Geometry check sheet. Reference: the model listing, model coordinates, mm. Face numbers are marked on the shaded views. A direction names the side the tool comes from. Give positions to 0.01 mm unless a question says otherwise; leave off trailing zeros. Write each loop counter-clockwise with the first axis right and the second up, starting at its lowest first coordinate (ties: lowest second). Pieces come first, ordered by that corner, then holes. Notation, with made-up numbers: M 39,81 L 86,81 A13 cw 86,89 Z; hole C -33,2 d4. An arc over 180 degrees is marked long. One line per item, written item: value. Start each with the question number.
1. Release check for a two-part mould opening along X. For the marked faces 1, 2 and 3 record: pulls with the +X half, pulls with the -X half, needs draft (parallel to the pull), parting line crosses it, or undercut.
2. Cross-section at D-D on x = 15. Record the cut outline in (y, z), then the cut area to 3 significant figures.
3. Cross-section at B-B on z = -11. Record the cut outline in (x, y).
4. Tool access check on the marked faces 4 and 5. Record the directions out of +Z, -Z, +X, -X, +Y, -Y that give a thin tool (end or side, any length) a straight path to the whole face; none if there is none.
5. Scan lines: line 1 (Y direction, x = 38.75, z = -46.99) (1 decimal); line 2 (Z direction, x = -22, y = 27). Record each from-to range of solid material in increasing order.
6. Gauge pin test, flat end, axial feed: pin 1 (6 mm diameter, centred on x = -21, y = 5.5, fed in from -Z). Record the tip position at first contact, or that the pin passes through.
7. Cross-section at A-A on y = 6.35. Record the cut outline in (x, z) (3 decimals), then the cut area to 3 significant figures.
8. Cross-section at C-C on z = -42. Record the cut outline in (x, y), then the cut area to 3 significant figures.
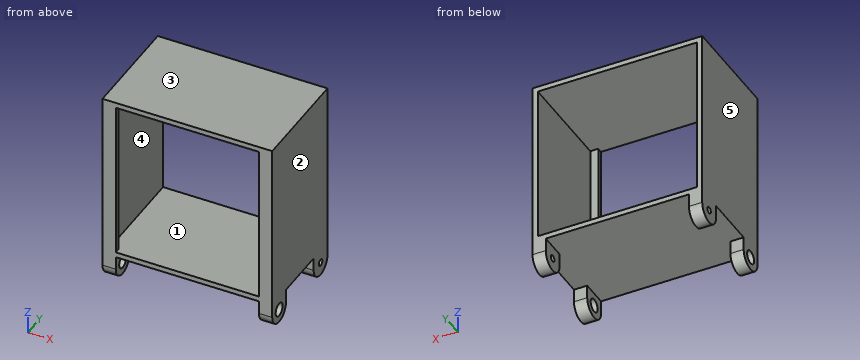
from build123d import *

# Parameters (mm, degrees)
SKETCH1_W           = 81.28
SKETCH1_H           = 81.28
SKETCH1_W_2         = 76.2
SKETCH1_H_2         = 76.2
BOSS_EXTRUDE1_DEPTH = 50.8
SKETCH2_W           = 3.81
SKETCH2_H           = 76.2
BOSS_EXTRUDE2_DEPTH = 2.54
SKETCH3_R           = 3.175
BOSS_EXTRUDE3_DEPTH = 6.35
SKETCH4_R           = 1.5875
BOSS_EXTRUDE4_DEPTH = 6.35


with BuildPart() as part:
    # Sketch1 → Boss-Extrude1 (new body)
    with BuildSketch(Plane(origin=(0, 0, 0), x_dir=(1, 0, 0), z_dir=(0, 1, 0))):
        Rectangle(SKETCH1_W, SKETCH1_H)
        Rectangle(SKETCH1_W_2, SKETCH1_H_2, mode=Mode.SUBTRACT)
    extrude(amount=BOSS_EXTRUDE1_DEPTH)

    # Sketch2 → Boss-Extrude2 (add)
    with BuildSketch(Plane(origin=(0, 0, 0), x_dir=(1, 0, 0), z_dir=(0, 1, 0))):
        with Locations((-36.195, 0)):
            Rectangle(SKETCH2_W, SKETCH2_H)
        with Locations((36.195, 0)):
            Rectangle(SKETCH2_W, SKETCH2_H)
    extrude(amount=BOSS_EXTRUDE2_DEPTH)

    # Sketch3 → Boss-Extrude3 (add)
    with BuildSketch(Plane(origin=(40.64, 0, 0), x_dir=(0, 0, -1), z_dir=(1, 0, 0))):
        with BuildLine():
            Line((46.99, 12.7), (40.64, 12.7))
            Line((40.64, 12.7), (40.64, 0))
            Line((40.64, 0), (46.99, 0))
            ThreePointArc((46.99, 0), (53.34, 6.35), (46.99, 12.7))
        make_face()
        with Locations((46.99, 6.35)):
            Circle(SKETCH3_R, mode=Mode.SUBTRACT)
    boss_extrude3 = extrude(amount=-BOSS_EXTRUDE3_DEPTH)

    # Sketch4 → Boss-Extrude4 (add)
    with BuildSketch(Plane(origin=(40.64, 0, 0), x_dir=(0, 0, -1), z_dir=(1, 0, 0))):
        with BuildLine():
            Line((46.99, 50.8), (40.64, 50.8))
            Line((40.64, 50.8), (40.64, 38.1))
            Line((40.64, 38.1), (46.99, 38.1))
            ThreePointArc((46.99, 38.1), (53.34, 44.45), (46.99, 50.8))
        make_face()
        with Locations((46.99, 44.45)):
            Circle(SKETCH4_R, mode=Mode.SUBTRACT)
    boss_extrude4 = extrude(amount=-BOSS_EXTRUDE4_DEPTH)

    # Mirror1: Boss-Extrude3, Boss-Extrude4 across plane
    add(boss_extrude3.mirror(Plane.ZY))
    add(boss_extrude4.mirror(Plane.ZY))


solid = part.part
Report:
1. face 1: undercut
1. face 2: pulls with the +X half
1. face 3: needs draft
2. outline: M 0,-40.64 L 50.8,-40.64 L 50.8,-38.1 L 0,-38.1 Z; M 0,38.1 L 50.8,38.1 L 50.8,40.64 L 0,40.64 Z
2. area: 258 mm^2
3. outline: M -40.64,0 L -34.29,0 L -34.29,2.54 L -38.1,2.54 L -38.1,50.8 L -40.64,50.8 Z; M 34.29,0 L 40.64,0 L 40.64,50.8 L 38.1,50.8 L 38.1,2.54 L 34.29,2.54 Z
4. face 4: +Y
4. face 5: +Z, -Z, -X, +Y, -Y
5. line 1: y = 0 to 3.2, 9.5 to 12.7, 38.1 to 42.9, 46 to 50.8
5. line 2: z = -40.64 to -38.1, 38.1 to 40.64
6. pin 1: stops at z = -40.64
7. outline: M -40.64,-53.34 L -34.29,-53.34 L -34.29,-50.165 L -40.64,-50.165 Z; M -40.64,-43.815 L -34.29,-43.815 L -34.29,-40.64 L 34.29,-40.64 L 34.29,-43.815 L 40.64,-43.815 L 40.64,40.64 L -40.64,40.64 Z; M 34.29,-53.34 L 40.64,-53.34 L 40.64,-50.165 L 34.29,-50.165 Z; hole M -38.1,-38.1 L 38.1,-38.1 L 38.1,38.1 L -38.1,38.1 Z
7. area: 881 mm^2
8. outline: M -40.64,0 L -34.29,0 L -34.29,12.7 L -40.64,12.7 Z; M -40.64,38.1 L -34.29,38.1 L -34.29,50.8 L -40.64,50.8 Z; M 34.29,0 L 40.64,0 L 40.64,12.7 L 34.29,12.7 Z; M 34.29,38.1 L 40.64,38.1 L 40.64,50.8 L 34.29,50.8 Z
8. area: 323 mm^2
